The listing builds one solid part. Answer for the finished solid, in the listing's coordinates (mm). A direction names the side the tool comes from. Coordinates: 2 decimals unless noted, no trailing zeros. Loops run counter-clockwise (first coordinate to the right, second up) from the corner with the lowest first, then second, coordinate; pieces in that order, holes last. Notation, with made-up numbers: M 80.25,12 L 107.25,12 A22 cw 107.25,33 Z; hole C 28.25,-39 d4. An arc over 180 degrees is marked long. Return JSON: item names as keys, results as strings. Group by question number.
1. Section D-D (x = -10) is taken. Write down the section's boundary in (y, z), then the cut area to 3 significant figures.
2. Straight lines are drawn through the part: L1, parallel to Z at x = 23, y = 42.1; L2, parallel to Z at x = 25, y = 14; L3, parallel to X at y = 27.5, z = 9. For each, find the intervals that lie inside material, in ascending order. Write a range as from..to.
3. The mould has two halves that part along X. Classify faces 4 (the face through (-23, 40, 12)), 5 (the face through (0, 0, 0)), 6 (the face through (-29, 22, 0)), 7 (the face through (29, 22, 0)): pulls with the +X half, pulls with the -X half, needs draft (parallel to the pull), parting line crosses it, or undercut.
4. Section A-A (z = 9) is taken. Write down the section's boundary in (x, y), then the cut area to 3 significant figures.
5. Which of the six approach directions +Z, -Z, +X, -X, +Y, -Y give full straight-line access (tool end or side, diameter ignored) to faces 1 (the face through (-10, 16, 5)), 2 (the face through (-3.47, 8.88, -10.07)), 3 (the face through (26, 40, -9))?
6. Section C-C (y = 24.5) is taken. Write down the section's boundary in (x, z), then the cut area to 3 significant figures.
7. Section B-B (x = -23) is taken. Write down the section's boundary in (y, z).
8. Given P1, Ø4.5, axis at x = -24.5, z = 10, coming from the +Y side; P2, Ø1, axis at x = 14.5, y = 20.5, coming from the +Z side; P3, Ø16, axis at x = 5, y = 22.5, coming from the -Z side, each flat-ended and moving along its own axis, determine where each tip first touches the part or whether it passes through.
```python
from build123d import *

# Parameters (mm, degrees)
SZKIC1_W                                             = 58
SZKIC1_H                                             = 30
DODANIE_WYCI_GNI_CIE1_DEPTH                          = 45
SZKIC3_R                                             = 12.5
WYTNIJ_WYCI_GNI_CIE2_DEPTH                           = 62.36774397
SZKIC4_R                                             = 16
WYTNIJ_WYCI_GNI_CIE3_DEPTH                           = 10
POG_BIENIE_WALCOWE_POD_M5_WKR_T_DO_CZ_CI_D           = 5.5
POG_BIENIE_WALCOWE_POD_M5_WKR_T_DO_CZ_CI_CBORE_D     = 9
POG_BIENIE_WALCOWE_POD_M5_WKR_T_DO_CZ_CI_CBORE_DEPTH = 5


with BuildPart() as part:
    # Szkic1 → Dodanie-wyciągnięcie1 (new body)
    with BuildSketch(Plane(origin=(0, 0, 0), x_dir=(1, 0, 0), z_dir=(0, 1, 0))):
        Rectangle(SZKIC1_W, SZKIC1_H)
    extrude(amount=DODANIE_WYCI_GNI_CIE1_DEPTH)

    # Szkic3 → Wytnij-wyciągnięcie2 (cut, through all)
    with BuildSketch(Plane.XY.offset(15)):
        with Locations((0, 24.5)):
            Circle(SZKIC3_R)
    extrude(amount=-WYTNIJ_WYCI_GNI_CIE2_DEPTH, mode=Mode.SUBTRACT)

    # Szkic4 → Wytnij-wyciągnięcie3 (cut)
    with BuildSketch(Plane.XY.offset(15)):
        with Locations((0, 24.5)):
            Circle(SZKIC4_R)
    wytnij_wyci_gni_cie3 = extrude(amount=-WYTNIJ_WYCI_GNI_CIE3_DEPTH, mode=Mode.SUBTRACT)

    # Lustro1: Wytnij-wyciągnięcie3 across plane
    add(wytnij_wyci_gni_cie3.mirror(Plane.XY), mode=Mode.SUBTRACT)

    # Pogłębienie walcowe pod M5 Wkręt do części metalowych z łbem sześciokątnym1 (through all)
    with Locations(Plane(origin=(0, 45, 0), x_dir=(1, 0, 0), z_dir=(0, 1, 0))):
        with Locations((-23, -9), (-23, 9), (23, -9), (23, 9)):
            CounterBoreHole(POG_BIENIE_WALCOWE_POD_M5_WKR_T_DO_CZ_CI_D / 2, POG_BIENIE_WALCOWE_POD_M5_WKR_T_DO_CZ_CI_CBORE_D / 2, POG_BIENIE_WALCOWE_POD_M5_WKR_T_DO_CZ_CI_CBORE_DEPTH)


solid = part.part
```
Worked out:
{
 "1": {"outline": "M 0,-15 L 12.01,-15 L 12.01,-5 L 17,-5 L 17,5 L 12.01,5 L 12.01,15 L 0,15 Z; M 32,-5 L 36.99,-5 L 36.99,-15 L 45,-15 L 45,15 L 36.99,15 L 36.99,5 L 32,5 Z", "area": "700 mm^2"},
 "2": {"L1": "-15..-13.5, -4.5..4.5, 13.5..15", "L2": "-15..-10.89, -7.11..7.11, 10.89..15", "L3": "-29..-25.75, -20.25..-15.72, 15.72..20.25, 25.75..29"},
 "3": {"face 4": "undercut", "face 5": "needs draft", "face 6": "pulls with the -X half", "face 7": "pulls with the +X half"},
 "4": {"outline": "M -29,0 L -25.75,0 L -25.75,40 L -27.5,40 L -27.5,45 L -29,45 Z; M -20.25,0 L 20.25,0 L 20.25,40 L 18.5,40 L 18.5,45 L -18.5,45 L -18.5,40 L -20.25,40 Z; M 25.75,0 L 29,0 L 29,45 L 27.5,45 L 27.5,40 L 25.75,40 Z; hole C 0,24.5 d32", "area": "1,280 mm^2"},
 "5": {"face 1": "+Z", "face 2": "-Z", "face 3": "+Y"},
 "6": {"outline": "M -29,-15 L -16,-15 L -16,-5 L -12.5,-5 L -12.5,5 L -16,5 L -16,15 L -29,15 Z; M 12.5,-5 L 16,-5 L 16,-15 L 29,-15 L 29,15 L 16,15 L 16,5 L 12.5,5 Z; hole C -23,-9 d5.5; hole C -23,9 d5.5; hole C 23,-9 d5.5; hole C 23,9 d5.5", "area": "755 mm^2"},
 "7": {"outline": "M 0,-15 L 45,-15 L 45,-13.5 L 40,-13.5 L 40,-11.75 L 0,-11.75 Z; M 0,-6.25 L 40,-6.25 L 40,-4.5 L 45,-4.5 L 45,4.5 L 40,4.5 L 40,6.25 L 0,6.25 Z; M 0,11.75 L 40,11.75 L 40,13.5 L 45,13.5 L 45,15 L 0,15 Z"},
 "8": {"P1": "y = 40", "P2": "z = 5", "P3": "z = -5"}
}
